Autodesk Inventor part; units mm, degrees
ref_plane "YZ Plane" through (0, 0, 0) normal (1, 0, 0) x (0, 1, 0)
ref_plane "XZ Plane" through (0, 0, 0) normal (0, 1, 0) x (-1, 0, 0)
ref_plane "XY Plane" through (0, 0, 0) normal (0, 0, 1) x (1, 0, 0)
sketch "Sketch1" plane through (0, 0, 0) normal (0, 0, 1) x (1, 0, 0)
  line L0 (0, 23) -> (-1, 23)
  line L1 (-1, 23) -> (-1, 13)
  line L2 (-1, 13) -> (-2, 13)
  line L3 (-2, 13) -> (-2, 10)
  line L4 (-2, 10) -> (-1.5, 10)
  line L5 (-1.5, 10) -> (-1.5, 0)
  line L6 (-1.5, 0) -> (0, 0)
  line L7 (0, 0) -> (0, 23)
  dimension "d0" = 1
  dimension "d1" = 1.5
  dimension "d2" = 2
  dimension "d3" = 10
  dimension "d4" = 10
  dimension "d5" = 3
revolve "Revolution1" add sketch "Sketch1" angle 360 about axis through (0, 0, 0) along (0, 1, 0)
thread "Thread1"
properties part number "Fitting-1" material "Brass"
Geometry check sheet. Reference: the model listing, model coordinates, mm. A direction names the side the tool comes from. Give positions to 0.01 mm unless a question says otherwise; leave off trailing zeros. Loops run counter-clockwise (first coordinate to the right, second up) from the corner with the lowest first, then second, coordinate; pieces in that order, holes last. Notation, with made-up numbers: M 52.5,-34.75 L 102.5,-34.75 A12 ccw 102.5,-24.75 Z; hole C 44,-16 d5. An arc over 180 degrees is marked long. Write item = value, one per line. Start each with the question number.
1. Section check D-D, the plane y = 9.75. Enter the section's corners in (x, z).
2. Section check C-C, the plane y = 14. Enter the section's corners in (x, z).
3. Go/stop test with flat-tipped pins: P1, Ø1.5, axis at x = 0, y = 6.5, coming from the +Z side; P2, Ø1, axis at y = 13, z = 1, coming from the +X side. Record where each tip stops, or that it passes through.
4. Thickness scan on probe 1 along Y at (x, z) = (-1.05, -1.15); probe 2 along Y at (x, z) = (0.75, 1.15); probe 3 along Z at (x, y) = (-1.1, 11.5). Record the ranges inside material, lowest first.
5. Section check A-A, the plane z = 0. Enter the section's corners in (x, y), plus the area to 3 significant figures.
6. Section check B-B, the plane x = 0. Enter the section's corners in (y, z), plus the area to 3 significant figures.
7. Tool access check on faces 1 (the face through (1.5, 4.93, -0.07)), 2 (the face through (0, 11, 2)), 3 (the face through (-1, 13, -1)). Record the directions out of +Z, -Z, +X, -X, +Y, -Y that give a thin tool (end or side, any length) a straight path to the whole face; none if there is none.
Values follow:
q1.outline = C 0,0 d3
q2.outline = C 0,0 d2
q3.P1 = 1.5
q3.P2 = 1.94
q4.probe_1 = 10 to 13
q4.probe_2 = 0 to 13
q4.probe_3 = -1.67 to 1.67
q5.outline = M -2,10 L -1.5,10 L -1.5,0 L 1.5,0 L 1.5,10 L 2,10 L 2,13 L 1,13 L 1,23 L -1,23 L -1,13 L -2,13 Z
q5.area = 62.0 mm^2
q6.outline = M 0,-1.5 L 10,-1.5 L 10,-2 L 13,-2 L 13,-1 L 23,-1 L 23,1 L 13,1 L 13,2 L 10,2 L 10,1.5 L 0,1.5 Z
q6.area = 62.0 mm^2
q7.face_1 = -Y
q7.face_2 = +Y, -Y
q7.face_3 = +Y
